from build123d import *

# Parameters (mm, degrees)
ESQUISSE1_R           = 1.75
BOSS_EXTRU_1_DEPTH    = 1.9
ESQUISSE2_W           = 35.7
ESQUISSE2_H           = 1.9
BOSS_EXTRU_2_DEPTH    = 21.4
CONG_1_R              = 2
CONG_2_R              = 0.2
CONG_3_R              = 2
BOSS_EXTRU_3_DEPTH    = 1.85
TROU_TARAUD_M41_D     = 3.3
BOSS_EXTRU_4_DEPTH    = 1.85
CONG_4_R              = 3
ESQUISSE7_W           = 8
ESQUISSE7_H           = 6.3
BOSS_EXTRU_5_DEPTH    = 1.85
CONG_5_R              = 1
CONG_6_R              = 2
CONG_4_OF_SYM_TRIE1_R = 3
CONG_5_OF_SYM_TRIE1_R = 1
CONG_6_OF_SYM_TRIE1_R = 2


with BuildPart() as part:
    # Esquisse1 → Boss.-Extru.1 (new body)
    with BuildSketch(Plane.XY):
        with BuildLine():
            Line((25, 0), (2.5, 0))
            Line((2.5, 0), (2.5, 2.8))
            ThreePointArc((2.5, 2.8), (0, 5.3), (-2.5, 2.8))
            Line((-2.5, 2.8), (-2.5, 0))
            Line((-2.5, 0), (-25, 0))
            Line((-25, 0), (-25, 130.5))
            Line((-25, 130.5), (25, 130.5))
            Line((25, 130.5), (25, 0))
        make_face()
        with Locations(Location((-18.05, 18.95, 0), (0, 0, 180))):
            Circle(ESQUISSE1_R, mode=Mode.SUBTRACT)
        with Locations(Location((18.05, 18.95, 0), (0, 0, 180))):
            Circle(ESQUISSE1_R, mode=Mode.SUBTRACT)
        with Locations(Location((0, 115.25, 0), (0, 0, 180))):
            Circle(ESQUISSE1_R, mode=Mode.SUBTRACT)
        with BuildLine():
            Line((-17.85, 26), (-17.85, 28.7))
            Line((-17.85, 28.7), (17.85, 28.7))
            Line((17.85, 28.7), (17.85, 26))
            ThreePointArc((17.85, 26), (18.95, 24.9), (20.05, 26))
            Line((20.05, 26), (20.05, 45.9))
            ThreePointArc((20.05, 45.9), (18.585533906, 49.435533906), (15.05, 50.9))
            Line((15.05, 50.9), (-15.05, 50.9))
            ThreePointArc((-15.05, 50.9), (-18.585533906, 49.435533906), (-20.05, 45.9))
            Line((-20.05, 45.9), (-20.05, 26))
            ThreePointArc((-20.05, 26), (-18.95, 24.9), (-17.85, 26))
        make_face(mode=Mode.SUBTRACT)
        with BuildLine():
            Line((-13.65, 86.2), (-0.65, 86.2))
            Line((-0.65, 86.2), (-0.65, 87.2))
            ThreePointArc((-0.65, 87.2), (0, 87.85), (0.65, 87.2))
            Line((0.65, 87.2), (0.65, 86.2))
            Line((0.65, 86.2), (13.65, 86.2))
            ThreePointArc((13.65, 86.2), (17.185533906, 84.735533906), (18.65, 81.2))
            Line((18.65, 81.2), (18.65, 67.8))
            ThreePointArc((18.65, 67.8), (17.185533906, 64.264466094), (13.65, 62.8))
            Line((13.65, 62.8), (-13.65, 62.8))
            ThreePointArc((-13.65, 62.8), (-17.185533906, 64.264466094), (-18.65, 67.8))
            Line((-18.65, 67.8), (-18.65, 81.2))
            ThreePointArc((-18.65, 81.2), (-17.185533906, 84.735533906), (-13.65, 86.2))
        make_face(mode=Mode.SUBTRACT)
    extrude(amount=BOSS_EXTRU_1_DEPTH)

    # Esquisse2 → Boss.-Extru.2 (add)
    with BuildSketch(Plane.XY.offset(1.9)):
        with Locations((0, 27.75)):
            Rectangle(ESQUISSE2_W, ESQUISSE2_H)
    extrude(amount=BOSS_EXTRU_2_DEPTH)

    # Congé1
    cong_1_edges = [part.edges().sort_by_distance(p)[0] for p in [
        (-17.85, 27.75, 23.3),
        (17.85, 27.75, 23.3),
    ]]
    fillet(cong_1_edges, radius=CONG_1_R)

    # Congé2
    cong_2_edges = [part.edges().sort_by_distance(p)[0] for p in [
        (0, 26.8, 1.9),
    ]]
    fillet(cong_2_edges, radius=CONG_2_R)

    # Congé3
    cong_3_edges = [part.edges().sort_by_distance(p)[0] for p in [
        (0, 28.7, 0),
    ]]
    fillet(cong_3_edges, radius=CONG_3_R)

    # Esquisse3 → Boss.-Extru.3 (add)
    with BuildSketch(Plane(origin=(0, 28.7, 0), x_dir=(1, 0, 0), z_dir=(0, 1, 0))):
        Polygon((6.12222325, -14.05), (7.998611625, -17.3), (11.751388375, -17.3), (13.62777675, -14.05), (11.751388375, -10.8), (7.998611625, -10.8), align=None)
        Polygon((-6.12222325, -14.05), (-7.998611625, -10.8), (-11.751388375, -10.8), (-13.62777675, -14.05), (-11.751388375, -17.3), (-7.998611625, -17.3), align=None)
    extrude(amount=BOSS_EXTRU_3_DEPTH)

    # Trou taraudé M41 (through all)
    with Locations(Plane(origin=(0, 30.55, 0), x_dir=(-1, 0, 0), z_dir=(0, 1, 0))):
        with Locations((-9.875, 14.05), (9.875, 14.05)):
            Hole(TROU_TARAUD_M41_D / 2)

    # Esquisse6 → Boss.-Extru.4 (add)
    with BuildSketch(Plane.ZY.offset(25)):
        with BuildLine():
            Line((13.4, 130.5), (13.4, 56))
            Line((13.4, 56), (29.6, 26.5))
            Line((29.6, 26.5), (29.6, 19.3))
            Line((29.6, 19.3), (27.05, 19.3))
            ThreePointArc((27.05, 19.3), (26.4, 18.65), (27.05, 18))
            Line((27.05, 18), (29.6, 18))
            Line((29.6, 18), (29.6, 11.3))
            Line((29.6, 11.3), (32.4, 11.3))
            Line((32.4, 11.3), (32.4, 5))
            Line((32.4, 5), (29.6, 5))
            Line((29.6, 5), (29.6, 0))
            Line((29.6, 0), (0, 0))
            Line((0, 0), (0, 130.5))
            Line((0, 130.5), (13.4, 130.5))
        make_face()
    boss_extru_4 = extrude(amount=-BOSS_EXTRU_4_DEPTH)

    # Congé4
    cong_4_edges = [part.edges().sort_by_distance(p)[0] for p in [
        (-24.075, 130.5, 13.4),
        (-24.075, 56, 13.4),
        (-24.075, 26.5, 29.6),
        (-24.075, 0, 29.6),
    ]]
    fillet(cong_4_edges, radius=CONG_4_R)

    # Esquisse7 → Boss.-Extru.5 (add)
    with BuildSketch(Plane.XY.offset(32.4)):
        with Locations((-21, 8.15)):
            Rectangle(ESQUISSE7_W, ESQUISSE7_H)
    boss_extru_5 = extrude(amount=-BOSS_EXTRU_5_DEPTH)

    # Congé5
    cong_5_edges = [part.edges().sort_by_distance(p)[0] for p in [
        (-17, 5, 31.475),
        (-17, 11.3, 31.475),
    ]]
    fillet(cong_5_edges, radius=CONG_5_R)

    # Congé6
    cong_6_edges = [part.edges().sort_by_distance(p)[0] for p in [
        (-25, 8.15, 32.4),
    ]]
    fillet(cong_6_edges, radius=CONG_6_R)

    # Symétrie1: Boss.-Extru.4, Boss.-Extru.5 across plane
    add(boss_extru_4.mirror(Plane(origin=(0, 0, 0), x_dir=(0, 0, 1), z_dir=(1, 0, 0))))
    add(boss_extru_5.mirror(Plane(origin=(0, 0, 0), x_dir=(0, 0, 1), z_dir=(1, 0, 0))))

    # Congé4 of Symétrie1
    cong_4_of_sym_trie1_edges = [part.edges().sort_by_distance(p)[0] for p in [
        (24.075, 130.5, 13.4),
        (24.075, 56, 13.4),
        (24.075, 26.5, 29.6),
        (24.075, 0, 29.6),
    ]]
    fillet(cong_4_of_sym_trie1_edges, radius=CONG_4_OF_SYM_TRIE1_R)

    # Congé5 of Symétrie1
    cong_5_of_sym_trie1_edges = [part.edges().sort_by_distance(p)[0] for p in [
        (17, 5, 31.475),
        (17, 11.3, 31.475),
    ]]
    fillet(cong_5_of_sym_trie1_edges, radius=CONG_5_OF_SYM_TRIE1_R)

    # Congé6 of Symétrie1
    cong_6_of_sym_trie1_edges = [part.edges().sort_by_distance(p)[0] for p in [
        (25, 8.15, 32.4),
    ]]
    fillet(cong_6_of_sym_trie1_edges, radius=CONG_6_OF_SYM_TRIE1_R)


solid = part.part
CAD build for the part. Positions are in the model's coordinates, mm. A direction names the side the tool comes from. Give positions to 0.01 mm unless a question says otherwise; leave off trailing zeros. Write each loop counter-clockwise with the first axis right and the second up, starting at its lowest first coordinate (ties: lowest second). Pieces come first, ordered by that corner, then holes. Notation, with made-up numbers: (29.5, 73) -> (82.5, 73) arc R26 cw to (82.5, 101) -> close; hole circle Ø6 at (-39.5, -12.5). An arc over 180 degrees is marked (long way). Return JSON: item names as keys, results as strings.
Item 1: Tool access for faces 1 (the flat face through (22, 11.3, 31)), 2 (the flat face through (0, 26.8, 13)), 3 (the cylindrical face through (18.62, 49.4, 0.94)), 4 (the flat face through (22, 5, 31)), 5 (the flat face through (-20, 8, 30.55)): list every direction of +Z, -Z, +X, -X, +Y, -Y with a clear straight run to the whole face (end or side of a thin tool).
Answer below:
{"face 1": "+Z, +X, -X, +Y", "face 2": "+Z, -Y", "face 3": "+Z, -Z", "face 4": "+Z, +X, -X, -Y", "face 5": "+Y, -Y"}
Item 2: Band-saw the part on B-B (y = 71.5). List the corners of the cut face in (x, z), then the cut area to 3 significant figures.
Answer below:
{"outline": "(-25, 0) -> (-18.65, 0) -> (-18.65, 1.9) -> (-23.15, 1.9) -> (-23.15, 13.4) -> (-25, 13.4) -> close; (18.65, 0) -> (25, 0) -> (25, 13.4) -> (23.15, 13.4) -> (23.15, 1.9) -> (18.65, 1.9) -> close", "area": "66.7 mm2"}
Item 3: Band-saw the part on C-C (z = 7.5). List the corners of the cut face in (x, y).
Answer below:
{"outline": "(-25, 0) -> (-23.15, 0) -> (-23.15, 130.5) -> (-25, 130.5) -> close; (-17.85, 26.8) -> (17.85, 26.8) -> (17.85, 28.7) -> (-17.85, 28.7) -> close; (23.15, 0) -> (25, 0) -> (25, 130.5) -> (23.15, 130.5) -> close"}
Item 4: Band-saw the part on D-D (y = 14). List the corners of the cut face in (x, z), then the cut area to 3 significant figures.
Answer below:
{"outline": "(-25, 0) -> (25, 0) -> (25, 29.6) -> (23.15, 29.6) -> (23.15, 1.9) -> (-23.15, 1.9) -> (-23.15, 29.6) -> (-25, 29.6) -> close", "area": "197 mm2"}
Item 5: Drill centre lines: probe 1 along X at (y, z) = (29, 14); probe 2 along X at (y, z) = (23, 10); probe 3 along Y at (x, z) = (18, 1). Where is each one in solid material? Low to high.
Answer below:
{"probe 1": "x = -25 to -23.15, -13.6 to -11.52, -8.23 to -6.15, 6.15 to 8.23, 11.52 to 13.6, 23.15 to 25", "probe 2": "x = -25 to -23.15, 23.15 to 25", "probe 3": "y = 0 to 17.2, 20.7 to 25.45, 49.94 to 65.33, 83.67 to 130.5"}
Item 6: Band-saw the part on A-A (x = -4). List the corners of the cut face in (y, z).
Answer below:
{"outline": "(0, 0) -> (26.7, 0) arc R2 ccw to (28.7, 2) -> (28.7, 23.3) -> (26.8, 23.3) -> (26.8, 2.1) arc R0.2 cw to (26.6, 1.9) -> (0, 1.9) -> close; (50.9, 0) -> (62.8, 0) -> (62.8, 1.9) -> (50.9, 1.9) -> close; (86.2, 0) -> (130.5, 0) -> (130.5, 1.9) -> (86.2, 1.9) -> close"}
Item 7: Two-plate mould, pull along X, no slides. Class faces 6 (the flat face through (-8, 30.55, 13)), 7 (the flat face through (25, 52, 12)), 8 (the cylindrical face through (24.06, 129.6, 12.54)): +X half, -X half, draft (parallel to the pull), parting line (faces both ways), or undercut.
Answer below:
{"face 6": "undercut", "face 7": "+X half", "face 8": "draft"}
Item 8: Drop flat-ended pins along their axis: pin 1 (6 mm diameter, centred on x = -18, z = 22, fed in from +Y); pin 2 (0.8 mm diameter, centred on x = -21.5, z = 31.5, fed in from +Y); pin 3 (0.6 mm diameter, centred on x = -24.5, z = 28.5, fed in from -Y). Give the stop position or say it passes through.
Answer below:
{"pin 1": "stops at y = 28.7", "pin 2": "stops at y = 11.3", "pin 3": "stops at y = 0.46"}
